```python
from build123d import *

# Parameters (mm, degrees)
BOSS_EXTRUDE1_DEPTH = 1
SKETCH2_W           = 9
SKETCH2_H           = 7
BOSS_EXTRUDE2_DEPTH = 6
CUT_EXTRUDE1_DEPTH  = 6
SKETCH4_W           = 3
SKETCH4_H           = 2
CUT_EXTRUDE3_DEPTH  = 7
CUT_EXTRUDE5_DEPTH  = 6
CUT_EXTRUDE6_DEPTH  = 6
CUT_EXTRUDE7_DEPTH  = 6


with BuildPart() as part:
    # Sketch1 → Boss-Extrude1 (new body)
    with BuildSketch(Plane.XY):
        Polygon((0, 4), (5, 9), (9, 9), (9, 0), (0, 0), align=None)
    extrude(amount=BOSS_EXTRUDE1_DEPTH)

    # Sketch2 → Boss-Extrude2 (add)
    with BuildSketch(Plane.XY.offset(1)):
        with Locations((4.5, 3.5)):
            Rectangle(SKETCH2_W, SKETCH2_H)
    extrude(amount=BOSS_EXTRUDE2_DEPTH)

    # 3DSketch1 → Cut-Extrude1 (cut, along a direction that is not the sketch's normal)
    with BuildSketch(Plane(origin=(7, 7, 4), x_dir=(-0.7427813527082076, -0.3713906763541037, 0.5570860145311556), z_dir=(0, 0.8320502943378437, 0.554700196225229))):
        Polygon((0, 0), (2.414039396, 2.678136254), (5.385164807, 0), (1.485562705, -1.339068127), align=None)
    extrude(amount=CUT_EXTRUDE1_DEPTH, dir=(0, 1, 0), mode=Mode.SUBTRACT)

    # Sketch4 → Cut-Extrude3 (cut)
    with BuildSketch(Plane.XY.offset(7)):
        with Locations((5.5, 1)):
            Rectangle(SKETCH4_W, SKETCH4_H)
    extrude(amount=-CUT_EXTRUDE3_DEPTH, mode=Mode.SUBTRACT)

    # Sketch5 → Cut-Extrude5 (cut)
    with BuildSketch(Plane(origin=(0, 7, 0), x_dir=(1, 0, 0), z_dir=(0, 1, 0))):
        Polygon((0, -7), (0, -4), (2, -6), (2, -7), align=None)
    extrude(amount=-CUT_EXTRUDE5_DEPTH, mode=Mode.SUBTRACT)

    # 3DSketch4 → Cut-Extrude6 (cut, along a direction that is not the sketch's normal)
    with BuildSketch(Plane(origin=(3, 5, 7), x_dir=(-0.5144957554275265, -0.5144957554275265, -0.6859943405700355), z_dir=(0.7071067811865475, -0.7071067811865476, 0))):
        Polygon((0, 0), (1.028991511, -0.9701425), (1.714985851, -0.242535625), (5.144957554, -0.727606875), (5.830951895, 0), (0.685994341, 4.850712501), (0, 4.123105626), align=None)
    extrude(amount=-CUT_EXTRUDE6_DEPTH, dir=(0, -1, 0), mode=Mode.SUBTRACT)

    # 3DSketch5 → Cut-Extrude7 (cut, along a direction that is not the sketch's normal)
    with BuildSketch(Plane(origin=(0, 2, 3), x_dir=(0.7071067811865476, 0.7071067811865475, 0), z_dir=(-0.577350269189626, 0.577350269189626, 0.5773502691896256))):
        Polygon((0, 0), (1.414213562, 2.449489743), (5.656854249, 2.449489743), (7.071067812, 0), align=None)
    extrude(amount=CUT_EXTRUDE7_DEPTH, dir=(0, 1, 0), mode=Mode.SUBTRACT)


solid = part.part
```
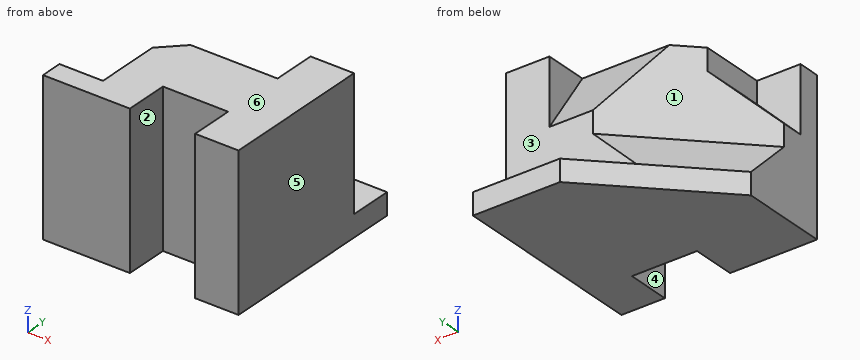
The listing builds one solid part. Answer for the finished solid, in the listing's coordinates (mm). Face numbers are marked on the shaded views. A direction names the side the tool comes from. Coordinates: 2 decimals unless noted, no trailing zeros. Write each loop counter-clockwise with the first axis right and the second up, starting at its lowest first coordinate (ties: lowest second). Pieces come first, ordered by that corner, then holes. Notation, with made-up numbers: M 1.5,-30 L 8.5,-30 A8 cw 8.5,-25 Z; hole C 54.5,-13 d10. An arc over 180 degrees is marked long. Use a Markdown table: item, result. Add a question column.
1. Section A-A (y = 1.5) is taken. Give the vertices of the cut face in (x, z).
2. Section D-D (x = 6.75) is taken. Give the vertices of the cut face in (y, z), plus the area to 3 significant figures.
3. Which of the six approach directions +Z, -Z, +X, -X, +Y, -Y give full straight-line access (tool end or side, diameter ignored) to the marked faces 1, 2 and 3?
4. Section C-C (y = 3.25) is taken. Give the vertices of the cut face in (x, z).
5. Section B-B (z = 4.75) is taken. Give the vertices of the cut face in (x, y), plus the area to 3 significant figures.
6. Straight lines are drawn through the part: line 1 along Y through (x, z) = (5, 1.5); line 2 along Y through (x, z) = (5.25, 5.5); line 3 along X through (y, z) = (3, 6.5). For each, find the intervals that lie inside material, in ascending order. Write a range as [from, to].
7. Given P1, Ø0.6, axis at y = 6.5, z = 6, coming from the -X side; P2, Ø4, axis at x = 4.5, z = 5, coming from the +Y side; P3, Ø2, axis at x = 6, y = 7.5, coming from the +Z side, each flat-ended and moving along its own axis, determine where each tip first touches the part or whether it passes through.
8. For a pull along X with two mould halves and no side action, classify the marked faces 4, 5 and 6 as +X half, -X half, draft (parallel to the pull), parting line (faces both ways), or undercut.
Data:
| question | item | result |
|---|---|---|
| 1 | outline | M 0,0 L 4,0 L 4,7 L 2,7 L 2,6 L 0,4 Z; M 7,0 L 9,0 L 9,7 L 7,7 Z |
| 2 | outline | M 2,0 L 9,0 L 9,1 L 7,1 L 7,4 L 5,7 L 2,7 Z |
| 2 | area | 34.0 mm2 |
| 3 | face 1 | +Z, -X, +Y |
| 3 | face 2 | +Z, -Z, -Y |
| 3 | face 3 | +Z, +X, -X, +Y |
| 4 | outline | M 0,0 L 9,0 L 9,7 L 2,7 L 2,6 L 1.25,5.25 L 1.25,3 L 0,1.75 Z |
| 5 | outline | M 0,0 L 4,0 L 4,2 L 7,2 L 7,0 L 9,0 L 9,7 L 7,7 L 7,6.5 L 4.5,6.5 L 0.75,2.75 L 0.75,1 L 0,1 Z |
| 5 | area | 42.3 mm2 |
| 6 | line 1 | y = [2, 7] |
| 6 | line 2 | y = [2, 6] |
| 6 | line 3 | x = [2, 9] |
| 7 | P1 | stops at x = 7 |
| 7 | P2 | stops at y = 7 |
| 7 | P3 | stops at z = 4.75 |
| 8 | face 4 | undercut |
| 8 | face 5 | +X half |
| 8 | face 6 | draft |
